The figure shows three views and two pictorial views of one solid part (mm, origin at its lowest corner). Answer the questions. A direction names the side the tool comes from. Give positions to 0.01 mm unless a question says otherwise; leave off trailing zeros. Write each loop counter-clockwise with the first axis right and the second up, starting at its lowest first coordinate (ties: lowest second). Pieces come first, ordered by that corner, then holes. Notation, with made-up numbers: (79, -3) - (123, -3) arc R24 cw to (123, 36) - close; hole circle Ø1 at (-15, 37). An arc over 180 degrees is marked (long way). Write each question's results on one line, items separated by ' | '. Start each with the question number.
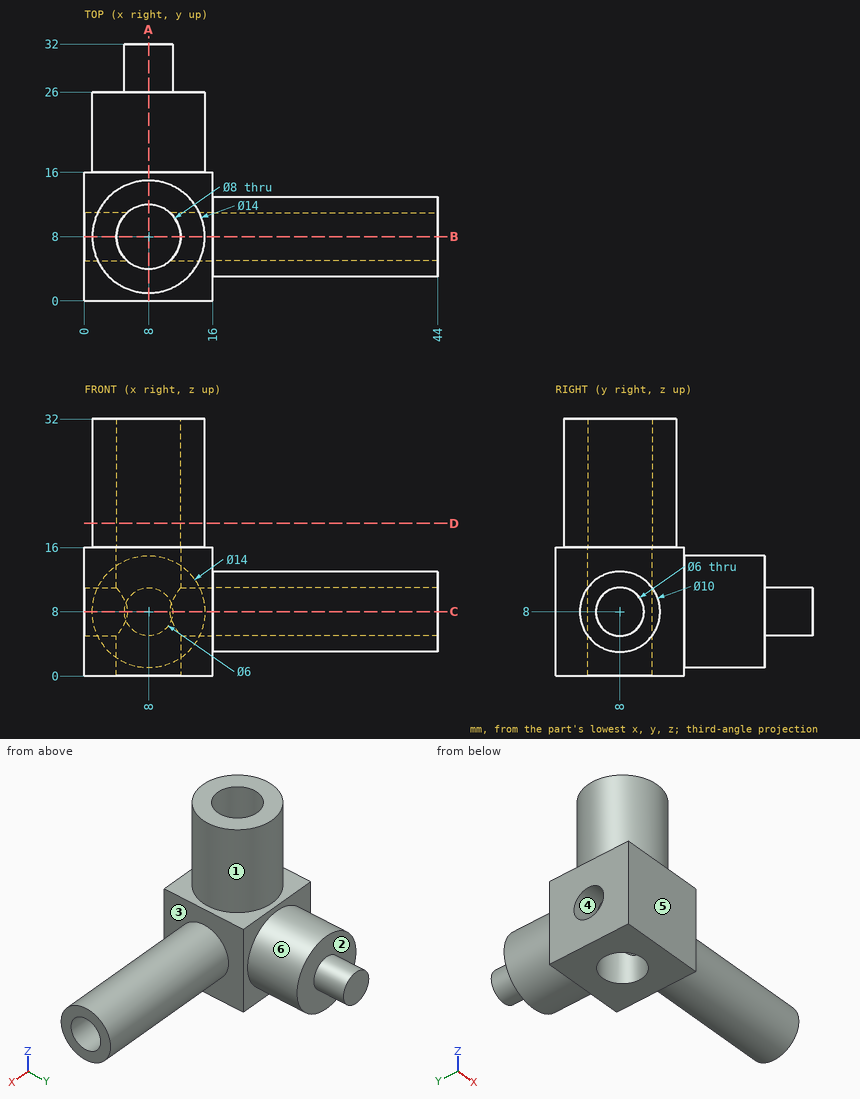
Q1. A cutting plane is placed at B-B, the plane y = 8. Write down the section's boundary in (x, z), and give its area (3 significant figures).
Q2. Consider L1, parallel to Z at x = 39, y = 8; L2, parallel to Y at x = 8, z = 3.5; L3, parallel to X at y = 10, z = 22. Determine where each line is inside the solid, lowest interval first.
Q3. A tool of negligible diameter and unlimited length cuts with its end or side. For the marked faces 1, 2 and 3, from which of +Z, -Z, +X, -X, +Y, -Y can it reach the whole face along a straight path? Write none if from no direction.
Q4. Given pin 1 (3 mm diameter, centred on x = 39, y = 3.5, fed in from +Z); pin 2 (4 mm diameter, centred on x = 5, z = 3.5, fed in from +Y); pin 3 (1 mm diameter, centred on x = 14.5, z = 20, fed in from -Y), each flat-ended and moving along its own axis, determine where each tip first touches the part or whether it passes through.
Q5. A cutting plane is placed at C-C, the plane z = 8. Write down the section's boundary in (x, y).
Q6. A cutting plane is placed at A-A, the plane x = 8. Write down the section's boundary in (y, z), and give its area (3 significant figures).
Q7. The mould has two halves that part along Y. Classify the marked faces 4, 5 and 6: pulls with the +Y half, pulls with the -Y half, needs draft (parallel to the pull), parting line crosses it, or undercut.
Q8. A cutting plane is placed at D-D, the plane z = 19. Write down the section's boundary in (x, y), and give its area (3 significant figures).
Result:
1) outline: (0, 0) - (4, 0) - (4, 5) - (0, 5) - close; (0, 11) - (4, 11) - (4, 32) - (1, 32) - (1, 16) - (0, 16) - close; (12, 0) - (16, 0) - (16, 3) - (44, 3) - (44, 5) - (12, 5) - close; (12, 11) - (44, 11) - (44, 13) - (16, 13) - (16, 16) - (15, 16) - (15, 32) - (12, 32) - close | area: 288 mm2
2) L1: z = 3 to 5, 11 to 13 | L2: y = 0 to 4, 12 to 26 | L3: x = 1.29 to 4.54, 11.46 to 14.71
3) face 1: +Z | face 2: +Y | face 3: +X
4) pin 1: stops at z = 12 | pin 2: stops at y = 26 | pin 3: stops at y = 4.39
5) outline: (0, 0) - (16, 0) - (16, 3) - (44, 3) - (44, 5) - (10.65, 5) arc R4 cw to (5.35, 5) - (0, 5) - close; (0, 11) - (5.35, 11) arc R4 cw to (10.65, 11) - (44, 11) - (44, 13) - (16, 13) - (16, 16) - (15, 16) - (15, 26) - (11, 26) - (11, 32) - (5, 32) - (5, 26) - (1, 26) - (1, 16) - (0, 16) - close
6) outline: (0, 0) - (4, 0) - (4, 32) - (1, 32) - (1, 16) - (0, 16) - close; (12, 0) - (16, 0) - (16, 1) - (26, 1) - (26, 5) - (32, 5) - (32, 11) - (26, 11) - (26, 15) - (16, 15) - (16, 16) - (15, 16) - (15, 32) - (12, 32) - close | area: 400 mm2
7) face 4: undercut | face 5: pulls with the -Y half | face 6: needs draft
8) outline: circle Ø14 at (8, 8); hole circle Ø8 at (8, 8) | area: 104 mm2
